```python
from build123d import *

# Parameters (mm, degrees)
CYLINDER010_R                               = 1.9
CYLINDER010_DEPTH                           = 14
BOX015_W                                    = 20
BOX015_H                                    = 13
BOX015_DEPTH                                = 19
CHAMFER004013007011015006009007001002_SIZE2 = 10
CHAMFER004013007011015006009007001002_SIZE  = 17
CHAMFER004013007011015006009007001003_SIZE  = 1


with BuildPart() as cylinder010:
    # Cylinder010 → Cylinder010 (new body)
    with BuildSketch(Plane(origin=(22, 7, 9.5), x_dir=(1, 0, 0), z_dir=(0, -1, 0))):
        Circle(CYLINDER010_R)
    extrude(amount=CYLINDER010_DEPTH)


with BuildPart() as supporter:
    # Box015 → Box015 (new body)
    with BuildSketch(Plane(origin=(9.5, -6.5, -3), x_dir=(1, 0, 0), z_dir=(0, 0, 1))):
        with Locations((10, 6.5)):
            Rectangle(BOX015_W, BOX015_H)
    extrude(amount=BOX015_DEPTH)

    # Chamfer004013007011015006009007001002
    chamfer004013007011015006009007001002_edges = [supporter.edges().sort_by_distance(p)[0] for p in [
        (29.5, 0, -3),
    ]]
    chamfer004013007011015006009007001002_side = supporter.faces().sort_by_distance((29.5, 0, 6.5))[0]
    chamfer(chamfer004013007011015006009007001002_edges, length=CHAMFER004013007011015006009007001002_SIZE, length2=CHAMFER004013007011015006009007001002_SIZE2, reference=chamfer004013007011015006009007001002_side)

    # Chamfer004013007011015006009007001003
    chamfer004013007011015006009007001003_edges = [supporter.edges().sort_by_distance(p)[0] for p in [
        (29.5, -6.5, 15),
        (29.5, 6.5, 15),
        (14.5, -6.5, -3),
        (24.5, -6.5, 5.5),
        (24.5, 6.5, 5.5),
        (14.5, 6.5, -3),
    ]]
    chamfer(chamfer004013007011015006009007001003_edges, length=CHAMFER004013007011015006009007001003_SIZE)

    # Cut028006004005011004003001006: cut Cylinder010
    add(cylinder010.part, mode=Mode.SUBTRACT)


solid = supporter.part
```
Here's how the part is built. I have some questions about the finished solid (model axes, mm). Round coordinates to 2 decimals unless told otherwise and drop trailing zeros. Order: outer loops, then holes, each group sorted by start corner. A loop starts at its lowest first (then second) coordinate and runs counter-clockwise, first axis right, second up. Notation, with made-up numbers: M 12.25,-36.75 L 62.25,-36.75 A19 ccw 62.25,-11.75 Z; hole C 70.5,9.5 d11. An arc over 180 degrees is marked long. Answer in a Markdown table with one row per item.
Item 1: Imagine slicing it at B-B, the plane z = 9.5. Write out the boundary of the cut face in (x, y), and give its area (3 significant figures).
A:
| item | result |
|---|---|
| outline | M 9.5,-6.5 L 20.1,-6.5 L 20.1,6.5 L 9.5,6.5 Z; M 23.9,-6.5 L 25.69,-6.5 L 26.85,-5.5 L 26.85,5.5 L 25.69,6.5 L 23.9,6.5 Z |
| area | 175 mm2 |
Item 2: Imagine slicing it at A-A, the plane x = 23. Write out the boundary of the cut face in (y, z).
A:
| item | result |
|---|---|
| outline | M -6.5,4.92 L -5.5,2.95 L 5.5,2.95 L 6.5,4.92 L 6.5,7.88 L -6.5,7.88 Z; M -6.5,11.12 L 6.5,11.12 L 6.5,16 L -6.5,16 Z |
Item 3: If I drill on L1, parallel to Z at x = 22, y = 3.75; L2, parallel to X at y = -0.25, z = 9.5; L3, parallel to Z at x = 20.75, y = 3.75 (3 decimals), over which ranges is the centre line in solid material (lowest first)? Write a range as from..to.
A:
| item | result |
|---|---|
| L1 | z = 1.25..7.6, 11.4..16 |
| L2 | x = 9.5..20.1, 23.9..26.85 |
| L3 | z = -0.875..8.069, 10.931..16 |
Item 4: I'm going to push flat-ended pins straight in: pin 1 (3 mm diameter, centred on y = 4.5, z = 8.5, fed in from +X); pin 2 (3 mm diameter, centred on x = 26, y = -4, fed in from -Z). Where does each tip first touch, or does it pass through?
A:
| item | result |
|---|---|
| pin 1 | stops at x = 27.15 |
| pin 2 | stops at z = 5.5 |
Item 5: Imagine slicing it at C-C, the plane y = -4.75. Write out the boundary of the cut face in (x, z), and give its area (3 significant figures).
A:
| item | result |
|---|---|
| outline | M 9.5,-3 L 19.5,-3 L 29.5,14 L 29.5,16 L 9.5,16 Z; hole C 22,9.5 d3.8 |
| area | 284 mm2 |
Item 6: Thinking about a two-plate mould opening in Z: for faces 1 (the face through (20.492, 0.091, 8.344)), 2 (the face through (24.43, -0.08, 5.38)), 3 (the face through (17, -6.5, 7)), which applies, +Z half, -Z half, draft (parallel to the pull), parting line (faces both ways), or undercut?
A:
| item | result |
|---|---|
| face 1 | undercut |
| face 2 | -Z half |
| face 3 | draft |
Item 7: Imagine slicing it at D-D, the plane z = 0. Write out the boundary of the cut face in (x, y), and give its area (3 significant figures).
A:
| item | result |
|---|---|
| outline | M 9.5,-6.5 L 20.1,-6.5 L 21.26,-5.5 L 21.26,5.5 L 20.1,6.5 L 9.5,6.5 Z |
| area | 152 mm2 |
